```python
from build123d import *

# Parameters (mm, degrees)
BOSS_EXTRUDE1_DEPTH = 10
BOSS_EXTRUDE2_START = 35
SKETCH2_R           = 2.5
BOSS_EXTRUDE2_DEPTH = 7
LPATTERN1_COUNT     = 3
LPATTERN1_PITCH     = 35
SHELL1_T            = -3
SKETCH3_W           = 8
SKETCH3_H           = 20
CUT_EXTRUDE1_DEPTH  = 20
BOSS_EXTRUDE3_START = 3
SKETCH5_R           = 2.5
BOSS_EXTRUDE3_DEPTH = 3
LPATTERN2_COUNT     = 2
LPATTERN2_PITCH     = 31
SKETCH6_W           = 28
SKETCH6_H           = 14
CUT_EXTRUDE2_DEPTH  = 3
BOSS_EXTRUDE4_START = 30
SKETCH7_R           = 2.5
BOSS_EXTRUDE4_DEPTH = 3
LPATTERN3_COUNT     = 2
LPATTERN3_PITCH     = 57


with BuildPart() as part:
    # Sketch1 → Boss-Extrude1 (new body, symmetric)
    with BuildSketch(Plane(origin=(0, 0, 0), x_dir=(1, 0, 0), z_dir=(0, 1, 0))):
        Polygon((-45, 0), (45, 0), (30, -100), (-30, -100), align=None)
    extrude(amount=BOSS_EXTRUDE1_DEPTH, both=True)

    # Sketch2 → Boss-Extrude2 (add, symmetric)
    with BuildSketch(Plane(origin=(0, 0, 0), x_dir=(0, 0, -1), z_dir=(1, 0, 0)).offset(BOSS_EXTRUDE2_START)):
        with BuildLine():
            Line((0, 10), (10, 10))
            ThreePointArc((10, 10), (20, 0), (10, -10))
            Line((10, -10), (0, -10))
            Line((0, -10), (0, 10))
        make_face()
        with Locations((10, 0)):
            Circle(SKETCH2_R, mode=Mode.SUBTRACT)
    boss_extrude2 = extrude(amount=BOSS_EXTRUDE2_DEPTH, both=True)

    # LPattern1: Boss-Extrude2 ×3
    with Locations(*[(-i * LPATTERN1_PITCH, 0, 0) for i in range(1, LPATTERN1_COUNT)]):
        add(boss_extrude2)

    # Shell1
    shell1_openings = [part.faces().sort_by_distance(p)[0] for p in [
        (0, 0, 100),
    ]]
    offset(amount=SHELL1_T, openings=shell1_openings, kind=Kind.INTERSECTION)

    # Sketch3 → Cut-Extrude1 (cut)
    with BuildSketch(Plane.XY):
        with Locations((35, 0)):
            Rectangle(SKETCH3_W, SKETCH3_H)
        Rectangle(SKETCH3_W, SKETCH3_H)
        with Locations((-35, 0)):
            Rectangle(SKETCH3_W, SKETCH3_H)
    extrude(amount=-CUT_EXTRUDE1_DEPTH, mode=Mode.SUBTRACT)

    # Sketch5 → Boss-Extrude3 (add)
    with BuildSketch(Plane(origin=(14.009779951, 0, 93.398533007), x_dir=(-0.988936353, 0, 0.148340453), z_dir=(-0.148340453, 0, -0.988936353)).offset(BOSS_EXTRUDE3_START)):
        with BuildLine():
            Line((44.502135879, 10), (54.502135879, 10))
            ThreePointArc((54.502135879, 10), (64.502135879, 0), (54.502135879, -10))
            Line((54.502135879, -10), (44.502135879, -10))
            Line((44.502135879, -10), (44.502135879, 10))
        make_face()
        with Locations((54.502135879, 0)):
            Circle(SKETCH5_R, mode=Mode.SUBTRACT)
    boss_extrude3 = extrude(amount=BOSS_EXTRUDE3_DEPTH)

    # LPattern2: Boss-Extrude3 ×2
    with Locations(*[Vector(-0.148340453, 0, -0.988936353) * (i * LPATTERN2_PITCH) for i in range(1, LPATTERN2_COUNT)]):
        add(boss_extrude3)

    # Sketch6 → Cut-Extrude2 (cut)
    with BuildSketch(Plane(origin=(-44.009779951, 0, 6.601466993), x_dir=(-0.148340453, 0, -0.988936353), z_dir=(0.988936353, 0, -0.148340453))):
        with Locations((-74.443421699, 0)):
            Rectangle(SKETCH6_W, SKETCH6_H)
    extrude(amount=CUT_EXTRUDE2_DEPTH, mode=Mode.SUBTRACT)

    # Sketch7 → Boss-Extrude4 (add)
    with BuildSketch(Plane(origin=(0, 0, 0), x_dir=(0, 0, -1), z_dir=(1, 0, 0)).offset(BOSS_EXTRUDE4_START)):
        with BuildLine():
            Line((-100, 10), (-110, 10))
            ThreePointArc((-110, 10), (-120, 0), (-110, -10))
            Line((-110, -10), (-100, -10))
            Line((-100, -10), (-100, 10))
        make_face()
        with Locations((-110, 0)):
            Circle(SKETCH7_R, mode=Mode.SUBTRACT)
    boss_extrude4 = extrude(amount=-BOSS_EXTRUDE4_DEPTH)

    # LPattern3: Boss-Extrude4 ×2
    with Locations(*[(-i * LPATTERN3_PITCH, 0, 0) for i in range(1, LPATTERN3_COUNT)]):
        add(boss_extrude4)


solid = part.part
```
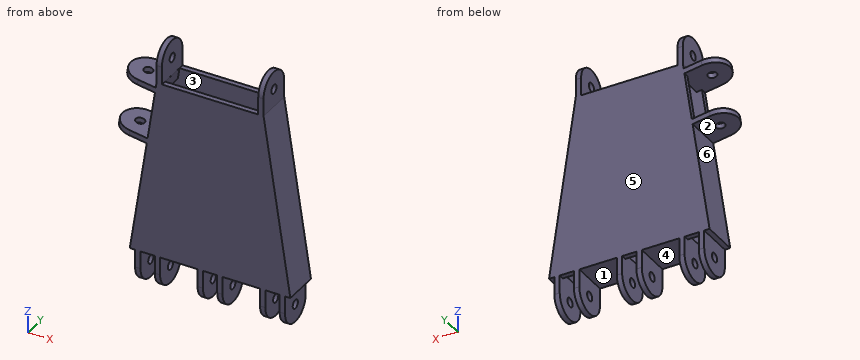
Design review of the part built by this model. Coordinates are the model's own, in mm. Face numbers are marked on the shaded views. A direction names the side the tool comes from. Coordinates: 2 decimals unless noted, no trailing zeros. Order: outer loops, then holes, each group sorted by start corner. A loop starts at its lowest first (then second) coordinate and runs counter-clockwise, first axis right, second up. Notation, with made-up numbers: (27.25, 9.25) - (55.25, 9.25) arc R21 ccw to (55.25, 26.25) - close; hole circle Ø9 at (65.25, 36.5). An arc over 180 degrees is marked (long way). Answer in a Markdown table with one row per item.
(1) For the marked faces 1, 2 and 3, list the 3-axis set-ups (+Z, -Z, +X, -X, +Y, -Y) from which the entire face can be reached by the end or side of a thin tool; tool diameter is ignored.
Checked values:
| item | result |
|---|---|
| face 1 | -Z, +Y, -Y |
| face 2 | -X, +Y, -Y |
| face 3 | none |
(2) Consider section B-B on x = 23.5. State the section outline as (y, z) points, plus the area to 3 significant figures.
Checked values:
| item | result |
|---|---|
| outline | (-10, 0) - (10, 0) - (10, 100) - (7, 100) - (7, 3) - (-7, 3) - (-7, 100) - (-10, 100) - close |
| area | 642 mm^2 |
(3) Consider section D-D on y = 0. Give the number of separate pieces and of enclosed holes in the cut face, plus the area to 3 significant figures.
Checked values:
| item | result |
|---|---|
| separate pieces | 15 |
| enclosed holes | 0 |
| area | 1,150 mm^2 |
(4) Clearance check with flat-ended pins moving along their axes: pin 1 (6 mm diameter, centred on y = -1, z = -6, fed in from -X); pin 2 (5 mm diameter, centred on y = 7, z = 72.5, fed in from +X); pin 3 (6.5 mm diameter, centred on y = 0, z = 110, fed in from +X); pin 4 (5 mm diameter, centred on x = 22.5, z = 105, fed in from +Y). State where each tip first meets the part, or that it passes through.
Checked values:
| item | result |
|---|---|
| pin 1 | x = -42 |
| pin 2 | x = 34.5 |
| pin 3 | x = 30 |
| pin 4 | through |
(5) Consider section C-C on z = 54. State the section outline as (x, y) points, plus the area to 3 significant figures.
Checked values:
| item | result |
|---|---|
| outline | (-36.9, -10) - (36.9, -10) - (36.9, 10) - (-36.9, 10) - close; hole (-33.87, -7) - (33.87, -7) - (33.87, 7) - (-33.87, 7) - close |
| area | 528 mm^2 |
(6) Wall thickness on line 1 along X through (y, z) = (-6.5, -12); line 2 along Y through (x, z) = (5, -10); line 3 along Y through (x, z) = (32, 61): over which ranges is each line inside the solid? List them lowest first. Write a range as from..to.
Checked values:
| item | result |
|---|---|
| line 1 | -42..-39, -31..-28, -7..-4, 4..7, 28..31, 39..42 |
| line 2 | -10..-2.5, 2.5..10 |
| line 3 | -10..-7, 7..10 |
(7) The part is to be moulded in two halves that separate along Z. For the marked faces 4, 5 and 6, say which applies: released by +Z, released by -Z, zero draft, split by the parting line, or undercut.
Checked values:
| item | result |
|---|---|
| face 4 | released by -Z |
| face 5 | zero draft |
| face 6 | undercut |
(8) Consider section A-A on z = 103. State the section outline as (x, y) points.
Checked values:
| item | result |
|---|---|
| outline | (-30, -10) - (-27, -10) - (-27, 10) - (-30, 10) - close; (27, -10) - (30, -10) - (30, 10) - (27, 10) - close |
